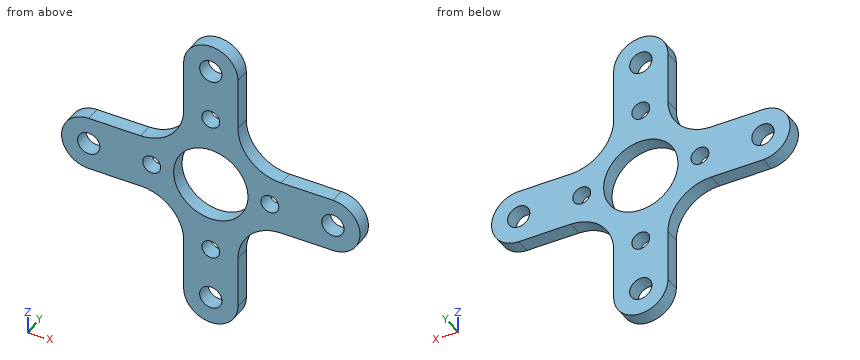
```python
from build123d import *

# Parameters (mm, degrees)
SKETCH1_R      = 1.5
SKETCH1_R_2    = 1.2
SKETCH1_R_3    = 5
EXTRUDE1_DEPTH = 2


with BuildPart() as part:
    # Sketch1 → Extrude1 (new body)
    with BuildSketch(Plane(origin=(0, 0, 0), x_dir=(1, 0, 0), z_dir=(0, 1, 0))):
        with BuildLine():
            Line((-1.80734609, 20.125232899), (-8.78234609, 20.125232899))
            ThreePointArc((-8.78234609, 20.125232899), (-12.883565421, 18.42645223), (-14.58234609, 14.325232899))
            Line((-14.58234609, 14.325232899), (-14.58234609, 7.350232899))
            ThreePointArc((-14.58234609, 7.350232899), (-18.23234609, 3.700232899), (-21.88234609, 7.350232899))
            Line((-21.88234609, 7.350232899), (-21.88234609, 14.325232899))
            ThreePointArc((-21.88234609, 14.325232899), (-23.581126759, 18.42645223), (-27.68234609, 20.125232899))
            Line((-27.68234609, 20.125232899), (-34.65734609, 20.125232899))
            ThreePointArc((-34.65734609, 20.125232899), (-38.30734609, 23.775232899), (-34.65734609, 27.425232899))
            Line((-34.65734609, 27.425232899), (-27.68234609, 27.425232899))
            ThreePointArc((-27.68234609, 27.425232899), (-23.581126759, 29.124013568), (-21.88234609, 33.225232899))
            Line((-21.88234609, 33.225232899), (-21.88234609, 40.200232899))
            ThreePointArc((-21.88234609, 40.200232899), (-18.23234609, 43.850232899), (-14.58234609, 40.200232899))
            Line((-14.58234609, 40.200232899), (-14.58234609, 33.225232899))
            ThreePointArc((-14.58234609, 33.225232899), (-12.883565421, 29.124013568), (-8.78234609, 27.425232899))
            Line((-8.78234609, 27.425232899), (-1.80734609, 27.425232899))
            ThreePointArc((-1.80734609, 27.425232899), (1.84265391, 23.775232899), (-1.80734609, 20.125232899))
        make_face()
        with Locations(Location((-18.23234609, 40.200232899, 0), (0, 0, 270))):
            Circle(SKETCH1_R, mode=Mode.SUBTRACT)
        with Locations(Location((-18.23234609, 7.350232899, 0), (0, 0, 270))):
            Circle(SKETCH1_R, mode=Mode.SUBTRACT)
        with Locations(Location((-34.65734609, 23.775232899, 0), (0, 0, 270))):
            Circle(SKETCH1_R, mode=Mode.SUBTRACT)
        with Locations(Location((-1.80734609, 23.775232899, 0), (0, 0, 270))):
            Circle(SKETCH1_R, mode=Mode.SUBTRACT)
        with Locations(Location((-26.18234609, 23.775232899, 0), (0, 0, 270))):
            Circle(SKETCH1_R_2, mode=Mode.SUBTRACT)
        with Locations(Location((-10.28234609, 23.775232899, 0), (0, 0, 270))):
            Circle(SKETCH1_R_2, mode=Mode.SUBTRACT)
        with Locations(Location((-18.23234609, 33.225232899, 0), (0, 0, 270))):
            Circle(SKETCH1_R_2, mode=Mode.SUBTRACT)
        with Locations(Location((-18.23234609, 14.325232899, 0), (0, 0, 270))):
            Circle(SKETCH1_R_2, mode=Mode.SUBTRACT)
        with Locations(Location((-18.23234609, 23.775232899, 0), (0, 0, 270))):
            Circle(SKETCH1_R_3, mode=Mode.SUBTRACT)
    extrude(amount=EXTRUDE1_DEPTH)


solid = part.part
```
The model under review builds one solid part; all positions refer to its coordinate system, in mm. Round coordinates to 2 decimals unless told otherwise and drop trailing zeros. Loops run counter-clockwise (first coordinate to the right, second up) from the corner with the lowest first, then second, coordinate; pieces in that order, holes last.
Item 1: For line 1 (Z direction, x = -18, y = 1.9); line 2 (Z direction, x = -34.5, y = 1.1); line 3 (X direction, y = 0.45, z = -24), list the stretches that pass through material, from the lowest coordinate up.
Determined:
line 1: z = -43.84 to -41.68, -38.72 to -34.4, -32.05 to -28.77, -18.78 to -15.5, -13.15 to -8.83, -5.87 to -3.71
line 2: z = -27.43 to -25.27, -22.28 to -20.13
line 3: x = -38.3 to -36.14, -33.17 to -27.36, -25 to -23.23, -13.24 to -11.46, -9.1 to -3.29, -0.32 to 1.84
Item 2: Take a section at A-A (x = -34). Write out the cut boundary in (y, z), then the cut area to 3 significant figures.
Determined:
outline: (0, -27.43) - (2, -27.43) - (2, -25.12) - (0, -25.12) - close; (0, -22.43) - (2, -22.43) - (2, -20.13) - (0, -20.13) - close
area: 9.21 mm2
Item 3: Clearance check with flat-ended pins moving along their axes: pin 1 Ø1 at (x, y) = (-32, 1.5) entering from -Z; pin 2 Ø0.6 at (y, z) = (1, -10.5) entering from +X. State where each tip first meets the part, or that it passes through.
Determined:
pin 1: stops at z = -27.43
pin 2: stops at x = -14.58
Item 4: Take a section at B-B (z = -15). Write out the cut boundary in (x, y).
Determined:
outline: (-21.92, 0) - (-19.22, 0) - (-19.22, 2) - (-21.92, 2) - close; (-17.24, 0) - (-14.54, 0) - (-14.54, 2) - (-17.24, 2) - close
Item 5: Take a section at C-C (y = 1.15). Give the number of separate pieces and of enclosed holes in the cut face, then the cut area to 3 significant figures.
Determined:
separate pieces: 1
enclosed holes: 9
area: 414 mm2
Item 6: Take a section at D-D (z = -30). Write out the cut boundary in (x, y), then the cut area to 3 significant figures.
Determined:
outline: (-22.86, 0) - (-13.6, 0) - (-13.6, 2) - (-22.86, 2) - close
area: 18.5 mm2
